from build123d import *

# Parameters (mm, degrees)
F1_DEPTH = 12.5


with BuildPart() as f1:
    # F0 (on Top) → F1 (new body, symmetric)
    with BuildSketch(Plane.XY):
        with BuildLine():
            ThreePointArc((39.889072, -2.976894), (39.972259, -1.48948), (40, 0))
            ThreePointArc((40, 0), (39.972259, 1.48948), (39.889072, 2.976894))
            ThreePointArc((39.889072, 2.976894), (35.453079, 6.251334), (38.501625, 10.845501))
            ThreePointArc((38.501625, 10.845501), (37.587705, 13.680806), (36.46531, 16.440231))
            ThreePointArc((36.46531, 16.440231), (31.176915, 18), (32.470313, 23.359769))
            ThreePointArc((32.470313, 23.359769), (30.641778, 25.711504), (28.643292, 27.920634))
            ThreePointArc((28.643292, 27.920634), (23.140354, 27.5776), (22.522602, 33.056503))
            ThreePointArc((22.522602, 33.056503), (20, 34.641016), (17.366471, 36.033397))
            ThreePointArc((17.366471, 36.033397), (12.312725, 33.828934), (9.858333, 38.766136))
            ThreePointArc((9.858333, 38.766136), (6.945927, 39.39231), (3.994997, 39.8))
            ThreePointArc((3.994997, 39.8), (0, 36), (-3.994997, 39.8))
            ThreePointArc((-3.994997, 39.8), (-6.945927, 39.39231), (-9.858333, 38.766136))
            ThreePointArc((-9.858333, 38.766136), (-12.312725, 33.828934), (-17.366471, 36.033397))
            ThreePointArc((-17.366471, 36.033397), (-20, 34.641016), (-22.522602, 33.056503))
            ThreePointArc((-22.522602, 33.056503), (-23.140354, 27.5776), (-28.643292, 27.920634))
            ThreePointArc((-28.643292, 27.920634), (-30.641778, 25.711504), (-32.470313, 23.359769))
            ThreePointArc((-32.470313, 23.359769), (-31.176915, 18), (-36.46531, 16.440231))
            ThreePointArc((-36.46531, 16.440231), (-37.587705, 13.680806), (-38.501625, 10.845501))
            ThreePointArc((-38.501625, 10.845501), (-35.453079, 6.251334), (-39.889072, 2.976894))
            ThreePointArc((-39.889072, 2.976894), (-40, 0), (-39.889072, -2.976894))
            ThreePointArc((-39.889072, -2.976894), (-35.453079, -6.251334), (-38.501625, -10.845501))
            ThreePointArc((-38.501625, -10.845501), (-37.587705, -13.680806), (-36.46531, -16.440231))
            ThreePointArc((-36.46531, -16.440231), (-31.176915, -18), (-32.470313, -23.359769))
            ThreePointArc((-32.470313, -23.359769), (-30.641778, -25.711504), (-28.643292, -27.920634))
            ThreePointArc((-28.643292, -27.920634), (-23.140354, -27.5776), (-22.522602, -33.056503))
            ThreePointArc((-22.522602, -33.056503), (-20, -34.641016), (-17.366471, -36.033397))
            ThreePointArc((-17.366471, -36.033397), (-12.312725, -33.828934), (-9.858333, -38.766136))
            ThreePointArc((-9.858333, -38.766136), (-6.945927, -39.39231), (-3.994997, -39.8))
            ThreePointArc((-3.994997, -39.8), (0, -36), (3.994997, -39.8))
            ThreePointArc((3.994997, -39.8), (6.945927, -39.39231), (9.858333, -38.766136))
            ThreePointArc((9.858333, -38.766136), (12.312725, -33.828934), (17.366471, -36.033397))
            ThreePointArc((17.366471, -36.033397), (20, -34.641016), (22.522602, -33.056503))
            ThreePointArc((22.522602, -33.056503), (23.140354, -27.5776), (28.643292, -27.920634))
            ThreePointArc((28.643292, -27.920634), (30.641778, -25.711504), (32.470313, -23.359769))
            ThreePointArc((32.470313, -23.359769), (31.176915, -18), (36.46531, -16.440231))
            ThreePointArc((36.46531, -16.440231), (37.587705, -13.680806), (38.501625, -10.845501))
            ThreePointArc((38.501625, -10.845501), (35.453079, -6.251334), (39.889072, -2.976894))
        make_face()
    extrude(amount=F1_DEPTH, both=True)


solid = f1.part
Work out the finished part from the listing and answer in its coordinate system (mm). Coordinates: 2 decimals unless noted, no trailing zeros. Write each loop counter-clockwise with the first axis right and the second up, starting at its lowest first coordinate (ties: lowest second). Pieces come first, ordered by that corner, then holes. Notation, with made-up numbers: (61, 41) - (108, 41) arc R19 ccw to (108, 62) - close; hole circle Ø11 at (43, 42). An arc over 180 degrees is marked (long way). One line per question, with ' | ' between items.
1) Consider probe 1 along Y at (x, z) = (26, 1); probe 2 along X at (y, z) = (1, -8.25); probe 3 along X at (y, z) = (-7, 8.5). Determine where each line is inside the solid, lowest interval first. Write a range as [from, to].
Checks:
probe 1: [-26.65, 26.65] | probe 2: [-39.99, 39.99] | probe 3: [-35.39, 35.39]
2) Find section B-B, the plane y = -20. Determine the outline of the cut face in (x, z).
Checks:
outline: (-30.64, -12.5) - (30.64, -12.5) - (30.64, 12.5) - (-30.64, 12.5) - close
3) Find section A-A, the plane y = -35. Determine the outline of the cut face in (x, z), and give its area (3 significant figures).
Checks:
outline: (-19.36, -12.5) - (-16.73, -12.5) - (-16.73, 12.5) - (-19.36, 12.5) - close; (-10.63, -12.5) - (10.63, -12.5) - (10.63, 12.5) - (-10.63, 12.5) - close; (16.73, -12.5) - (19.36, -12.5) - (19.36, 12.5) - (16.73, 12.5) - close | area: 663 mm2
4) Flat-ended cylindrical pins translate along their axes: P1, Ø1, axis at y = -14, z = 3, coming from the +X side; P2, Ø8, axis at x = -10, z = 7, coming from the -Y side; P3, Ø10, axis at x = 28.5, z = 8, coming from the -Y side. Find the tip coordinate at first contact, or state that the pin passes through.
Checks:
P1: x = 37.65 | P2: y = -39.55 | P3: y = -27.92
5) Find section C-C, the plane x = 0. Determine the outline of the cut face in (y, z).
Checks:
outline: (-36, -12.5) - (36, -12.5) - (36, 12.5) - (-36, 12.5) - close
6) The mould has two halves that part along X. Classify faces 1 (the face through (30.67, 25.68, 0.18)), 2 (the face through (-37.602, -13.642, 0.175)), 3 (the face through (23.21, 27.52, 0.18)): +X half, -X half, draft (parallel to the pull), parting line (faces both ways), or undercut.
Checks:
face 1: +X half | face 2: -X half | face 3: undercut
